Design review of the part built by this model. Coordinates are the model's own, in mm. A direction names the side the tool comes from. Coordinates: 2 decimals unless noted, no trailing zeros. Write each loop counter-clockwise with the first axis right and the second up, starting at its lowest first coordinate (ties: lowest second). Pieces come first, ordered by that corner, then holes.
Q1. Add section A-A, the plane x = 0.5. Give the boundary of the cut face in (y, z).
Q2. Add section B-B, the plane z = 2.5. Give the boundary of the cut face in (x, y).
Q3. Clearance check with a flat-ended pin moving along its axis: pin 1 Ø2 at (x, z) = (0, 2) entering from -Y. State where the tip first meets the part, or that it passes through.
Q4. Add section C-C, the plane y = 0. Give the boundary of the cut face in (x, z).
Q5. Machinability: for faces 1 (the face through (1, 2, 0)), 2 (the face through (-2, -1, 30)), 3 (the face through (-1.58, -2.55, 14.79)), which of the approach directions +Z, -Z, +X, -X, +Y, -Y give a long, thin tool a straight path to every point of the face, cutting with its end or side? Answer none if there is none.
Q6. To check wall thickness, follow probe 1 along Z at (x, y) = (-1.5, 2); probe 2 along X at (y, z) = (1.5, 9); probe 3 along Z at (x, y) = (1.5, 1). State the ranges of each line that lie inside material, in increasing order.
Q7. Add section D-D, the plane z = 30.5. Give the boundary of the cut face in (x, y), plus the area to 3 significant figures.
from build123d import *

# Parameters (mm, degrees)
BOSS_EXTRUDE1_DEPTH = 30
SKETCH2_R           = 2
BOSS_EXTRUDE2_DEPTH = 3
SKETCH3_R           = 1.6
BOSS_EXTRUDE3_DEPTH = 2


with BuildPart() as part:
    # Sketch1 → Boss-Extrude1 (new body)
    with BuildSketch(Plane.XY):
        Polygon((2.961597897, -1.796924567), (3.036981272, 1.666356731), (0.075383375, 3.463281298), (-2.961597897, 1.796924567), (-3.036981272, -1.666356731), (-0.075383375, -3.463281298), align=None)
    extrude(amount=BOSS_EXTRUDE1_DEPTH)

    # Sketch2 → Boss-Extrude2 (add)
    with BuildSketch(Plane.XY.offset(30)):
        Circle(SKETCH2_R)
    extrude(amount=BOSS_EXTRUDE2_DEPTH)

    # Sketch3 → Boss-Extrude3 (add)
    with BuildSketch(Plane(origin=(0, 0, 0), x_dir=(-1, 0, 0), z_dir=(0, 0, -1))):
        Circle(SKETCH3_R)
    extrude(amount=BOSS_EXTRUDE3_DEPTH)


solid = part.part
Here are the results:
1. outline: (-3.15, 0) - (-1.52, 0) - (-1.52, -2) - (1.52, -2) - (1.52, 0) - (3.21, 0) - (3.21, 30) - (1.94, 30) - (1.94, 33) - (-1.94, 33) - (-1.94, 30) - (-3.15, 30) - close
2. outline: (-3.04, -1.67) - (-0.08, -3.46) - (2.96, -1.8) - (3.04, 1.67) - (0.08, 3.46) - (-2.96, 1.8) - close
3. pin 1: stops at y = -3.46
4. outline: (-3, 0) - (-1.6, 0) - (-1.6, -2) - (1.6, -2) - (1.6, 0) - (3, 0) - (3, 30) - (2, 30) - (2, 33) - (-2, 33) - (-2, 30) - (-3, 30) - close
5. face 1: -Z
5. face 2: +Z
5. face 3: +Z, -Z, -X, -Y
6. probe 1: z = 0 to 30
6. probe 2: x = -2.97 to 3.03
6. probe 3: z = 0 to 33
7. outline: circle Ø4 at (0, 0)
7. area: 12.6 mm2
